Autodesk Inventor part; units mm, degrees
ref_plane "YZ Plane" through (0, 0, 0) normal (1, 0, 0) x (0, 1, 0)
ref_plane "XZ Plane" through (0, 0, 0) normal (0, 1, 0) x (-1, 0, 0)
ref_plane "XY Plane" through (0, 0, 0) normal (0, 0, 1) x (1, 0, 0)
sketch "Sketch1" plane through (0, 0, 0) normal (0, 0, 1) x (1, 0, 0)
  line L0 (-65.7184, 0) -> (65.7184, 0)
  line L1 (-36.2446, 59.05) -> (36.2446, 59.05)
  circle A0 centre (-30.5, 47) radius 8.55
  line L2 (0, 59.05) -> (0, 0) construction
  circle A1 centre (-30.5, 47) radius 6
  circle A2 centre (30.5, 47) radius 6
  arc A3 (-69.1825, 6) -> (-65.7184, 0) centre (-65.7184, 4) ccw
  arc A4 (-36.2446, 59.05) -> (-39.7087, 57.05) centre (-36.2446, 55.05) ccw
  line L3 (-69.1825, 6) -> (-39.7087, 57.05)
  arc A5 (65.7184, 0) -> (69.1825, 6) centre (65.7184, 4) ccw
  arc A6 (39.7087, 57.05) -> (36.2446, 59.05) centre (36.2446, 55.05) ccw
  line L4 (69.1825, 6) -> (39.7087, 57.05)
  line L5 (-65.7184, 3) -> (-30.5, 3)
  line L6 (-30.5, 3) -> (-30.5, 0)
  line L7 (-30.5, 0) -> (-65.7184, 0)
  line L8 (-65.7184, 0) -> (-65.7184, 3)
  line L9 (-30.5, 38.45) -> (0, 38.45) construction
  line L10 (-30.5, 3) -> (0, 3) construction
  line L11 (0, 38.45) -> (0, 3) construction
  line L12 (-60.5222, 9) -> (-47.5607, 31.45)
  line L13 (-47.5607, 31.45) -> (47.5607, 31.45)
  line L14 (47.5607, 31.45) -> (60.5222, 9)
  line L15 (60.5222, 9) -> (-60.5222, 9)
  circle A7 centre (30.5, 47) radius 9.55
  circle A8 centre (13.738, 5) radius 9.55
  circle A9 centre (13.738, 5) radius 6
  line L16 (-30.5, 47) -> (13.738, 5) construction
  circle A10 centre (13.738, 5) radius 13.05
  point P0 (-65.7184, 1.5)
  point P1 (-48.1092, 0)
  point P2 (-65.7184, 0)
  point P3 (-30.5, 0)
  point P4 (-30.5, 1.5)
  point P5 (0, 20.725)
  point P6 (0, 20.725)
  point P7 (0, 20.725)
  point P8 (25.7921, 0)
  point P9 (1.6838, 0)
  point P10 (26.1598, 9)
  point P11 (1.3161, 9)
  dimension "d1" = 17.1
  dimension "d3" = 3.5
  dimension "d7" = 12
  dimension "d10" = 4
  dimension "d11" = 13
  dimension "d12" = 60
  dimension "d17" = 3
  dimension "d22" = 44
  dimension "d40" = 6
  dimension "d41" = 6
  dimension "d43" = 6
  dimension "d44" = 19.1
  dimension "d45" = 61
  dimension "d46" = 6
  dimension "d49" = 19.1
  dimension "d51" = 5
  dimension "d52" = 61
  dimension "d54" = 26.1
extrude "Extrusion1" add sketch "Sketch1" along normal mid plane 30 contours A3 L3 A4 L1 A6 L4 A5 L0 A10 L15 L14 L13 L12 L6 L5 L8 | A10 L15 A8 L0 | L0 A8 A10 | A10 L15 A8 | L0 A8 L15 A10
extrude "Extrusion2" add sketch "Sketch1" along normal mid plane 20 contours A8 L15 A9 L0 | L0 A9 A8 | A8 L15 A9 | L0 A9 L15 A8 | A0 | A7
extrude "Extrusion3" add sketch "Sketch1" along normal blind 27.5 contours L8 L5 L6 L0
sketch "Sketch2" plane through (-65.7184, 3, 15) normal (0, 1, 0) x (1, 0, 0)
  line L0 (0, -12.5) -> (35.2184, -12.5)
  arc A0 (20.1092, -12.5) -> (15.1092, -12.5) centre (17.6092, -8.1699) ccw
  line L1 (35.2184, 0) -> (131.4367, 0) construction
  line L2 (35.2184, 0) -> (35.2184, -12.5) construction
  point P0 (65.7184, 15)
  point P1 (17.6092, -12.5)
  point P2 (17.6092, -3.1699)
  dimension "d21" = 5
  dimension "d25" = 5
extrude "Extrusion4" cut sketch "Sketch2" against normal through all
extrude "Extrusion6" add sketch "Sketch1" against normal blind 15 contours L8 L5 L6 L0
properties part number "EngineMount - Big hole"
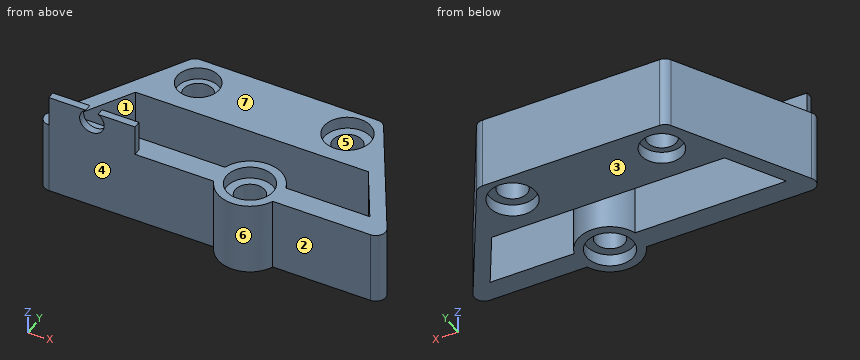
Read the model definition and answer for the solid it produces. Units are mm, in the model's axes. Face numbers are marked on the shaded views. A direction names the side the tool comes from. Coordinates: 2 decimals unless noted, no trailing zeros. Write each loop counter-clockwise with the first axis right and the second up, starting at its lowest first coordinate (ties: lowest second). Pieces come first, ordered by that corner, then holes. Notation, with made-up numbers: (73.5, 38.5) - (121.5, 38.5) arc R24 cw to (121.5, 72.5) - close; hole circle Ø10 at (-22.5, 44.5). An arc over 180 degrees is marked (long way). One line per question, with ' | ' between items.
Q1. For the marked faces 1, 2, 3 and 4, determine the directions among +Z, -Z, +X, -X, +Y, -Y from which every point of the face is accessible in a straight line to the end or side of a thin tool.
Result set:
face 1: +Z, -Z | face 2: +Z, -Z, +X, -Y | face 3: -Z, +X, -X, +Y, -Y | face 4: +Z, -Z, -X, -Y
Q2. Determine the mould class of the marked faces 5, 6 and 7 for opening direction X: +X half, -X half, draft (parallel to the pull), parting line (faces both ways), or undercut.
Result set:
face 5: undercut | face 6: parting line | face 7: draft
Q3. Find section D-D, the plane z = 20. Write down the section's boundary in (x, y), plus the area to 3 significant figures.
Result set:
outline: (-65.72, 0) - (-51.98, 0) - (-51.98, 3) - (-65.72, 3) - close; (-44.24, 0) - (-30.5, 0) - (-30.5, 3) - (-44.24, 3) - close | area: 82.5 mm^2
Q4. Find section C-C, the plane y = 47. Write down the section's boundary in (x, z).
Result set:
outline: (-45.51, -15) - (-39.05, -15) - (-39.05, -10) - (-36.5, -10) - (-36.5, 10) - (-39.05, 10) - (-39.05, 15) - (-45.51, 15) - close; (-24.5, -10) - (-21.95, -10) - (-21.95, -15) - (20.95, -15) - (20.95, -10) - (24.5, -10) - (24.5, 10) - (20.95, 10) - (20.95, 15) - (-21.95, 15) - (-21.95, 10) - (-24.5, 10) - close; (36.5, -10) - (40.05, -10) - (40.05, -15) - (45.51, -15) - (45.51, 15) - (40.05, 15) - (40.05, 10) - (36.5, 10) - close
Q5. Each of these flat-tipped pins is pushed along its axis until it touches: P1, Ø2, axis at x = -33.5, y = 7.5, coming from the +Z side; P2, Ø6, axis at y = 19.5, z = -0.5, coming from the +X side; P3, Ø1.5, axis at y = 30.5, z = 4.5, coming from the -X side; P4, Ø24, axis at x = 43, z = -5, coming from the +Y side. Where does it stop, or does it pass through?
Result set:
P1: z = 15 | P2: x = 63.12 | P3: x = -55.47 | P4: y = 59.05
Q6. Find section A-A, the plane x = 30.5. Write down the section's boundary in (y, z), plus the area to 3 significant figures.
Result set:
outline: (0, -15) - (9, -15) - (9, 15) - (0, 15) - close; (31.45, -15) - (37.45, -15) - (37.45, -10) - (41, -10) - (41, 10) - (37.45, 10) - (37.45, 15) - (31.45, 15) - close; (53, -10) - (56.55, -10) - (56.55, -15) - (59.05, -15) - (59.05, 15) - (56.55, 15) - (56.55, 10) - (53, 10) - close | area: 667 mm^2
Q7. Consider L1, parallel to Y at x = 30.5, z = 5; L2, parallel to X at y = 13, z = 5.5; L3, parallel to Y at x = -8.5, z = -8.5. Determine where each line is inside the solid, lowest interval first. Write a range as [from, to].
Result set:
L1: [0, 9], [31.45, 41], [53, 59.05] | L2: [-65.14, -58.21], [3.43, 24.05], [58.21, 65.14] | L3: [0, 9], [31.45, 59.05]
Q8. Find section B-B, the plane z = -8.5. Write down the section's boundary in (x, y).
Result set:
outline: (-69.18, 6) arc R4 ccw to (-65.72, 0) - (1.68, 0) arc R13.05 ccw to (25.79, 0) - (65.72, 0) arc R4 ccw to (69.18, 6) - (39.71, 57.05) arc R4 ccw to (36.24, 59.05) - (-36.24, 59.05) arc R4 ccw to (-39.71, 57.05) - close; hole (-60.52, 9) - (1.32, 9) arc R13.05 cw to (26.16, 9) - (60.52, 9) - (47.56, 31.45) - (-47.56, 31.45) - close; hole circle Ø12 at (-30.5, 47); hole circle Ø12 at (13.74, 5); hole circle Ø12 at (30.5, 47)
